Input: part model. Units: mm. Frame: model coordinates. Face numbers are marked on the shaded views. A direction names the side the tool comes from. Coordinates: 2 decimals unless noted, no trailing zeros. Loops run counter-clockwise (first coordinate to the right, second up) from the corner with the lowest first, then second, coordinate; pieces in that order, holes last. Notation, with made-up numbers: (86.25, -4) - (100.25, -4) arc R11 ccw to (100.25, 3) - close; hole circle Ø9 at (6.5, 27.25). An arc over 180 degrees is marked (long way). Write item = value, one per line. Start each with the question number.
from build123d import *

# Parameters (mm, degrees)
SKETCH_1_R          = 14
EXTRUDE_1_DEPTH     = 14
SKETCH_3_R          = 7.5
EXTRUDE_3_DEPTH     = 4
SKETCH_4_R          = 1.75
CUT_EXTRUDE_1_DEPTH = 27.758176321
SKETCH_5_R          = 1
CUT_EXTRUDE_2_DEPTH = 3
SKETCH_6_R          = 1.5
CUT_EXTRUDE_3_DEPTH = 3


with BuildPart() as part:
    # 草图1 → 凸台-拉伸1 (new body)
    with BuildSketch(Plane.XY):
        Circle(SKETCH_1_R)
    extrude(amount=EXTRUDE_1_DEPTH)

    # 草图3 → 凸台-拉伸3 (add)
    with BuildSketch(Plane.XY.offset(14)):
        Circle(SKETCH_3_R)
    extrude(amount=EXTRUDE_3_DEPTH)

    # 草图4 → 切除-拉伸1 (cut, through all)
    with BuildSketch(Plane.XY.offset(18)):
        Circle(SKETCH_4_R)
    extrude(amount=-CUT_EXTRUDE_1_DEPTH, mode=Mode.SUBTRACT)

    # 草图5 → 切除-拉伸2 (cut)
    with BuildSketch(Plane.XY.offset(18)):
        with Locations((0, -6)):
            Circle(SKETCH_5_R)
        with Locations((-6, 0)):
            Circle(SKETCH_5_R)
        with Locations((0, 6)):
            Circle(SKETCH_5_R)
        with Locations((6, 0)):
            Circle(SKETCH_5_R)
    extrude(amount=-CUT_EXTRUDE_2_DEPTH, mode=Mode.SUBTRACT)

    # 草图6 → 切除-拉伸3 (cut)
    with BuildSketch(Plane.XY):
        with Locations((0, 8)):
            Circle(SKETCH_6_R)
        with Locations((-8, 0)):
            Circle(SKETCH_6_R)
        with Locations((0, -8)):
            Circle(SKETCH_6_R)
        with Locations((8, 0)):
            Circle(SKETCH_6_R)
    extrude(amount=CUT_EXTRUDE_3_DEPTH, mode=Mode.SUBTRACT)


solid = part.part
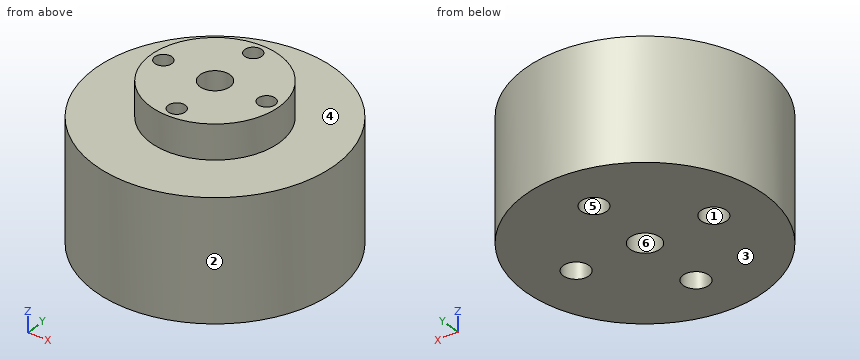
Item 1: Cut plane C-C on z = 1.75. Return loops of the section in (x, y), plus the area to 3 significant figures.
Item 2: Pull-direction query (Y, two-part tool) for the marked faces 1, 2 and 3; classes: pulls with the +Y half, pulls with the -Y half, needs draft (parallel to the pull), parting line crosses it, or undercut.
Item 3: Cut plane D-D on x = 9. Return loops of the section in (y, z), plus the area to 3 significant figures.
Item 4: Pin query (flat end, axial travel): pin 1 (6 mm diameter, centred on x = 8.5, z = 13.5, fed in from -Y); pin 2 (2.5 mm diameter, centred on x = 0, y = 8, fed in from -Z); pin 3 (1.6 mm diameter, centred on x = 0, y = -6, fed in from +Z). Return the tip coordinate at first contact, or that it passes through.
Item 5: Ray query, line 1 (Y direction, x = 0, z = 16.1); line 2 (Y direction, x = 0, z = 6.25); line 3 (Z direction, x = 6, y = 0). Return the intervals inside material, ascending.
Item 6: Cut plane A-A on x = 0. Return loops of the section in (y, z), plus the area to 3 significant figures.
Item 7: Access query for the marked faces 4, 5 and 6. Directions: +Z, -Z, +X, -X, +Y, -Y. A direction counts if a zero-diameter tool reaches every point of the face in a straight line with its end or side. Return the directions, or none.
Recorded:
q1.outline = circle Ø28 at (0, 0); hole circle Ø3 at (-8, 0); hole circle Ø3.5 at (0, 0); hole circle Ø3 at (0, -8); hole circle Ø3 at (0, 8); hole circle Ø3 at (8, 0)
q1.area = 578 mm²
q2.face_1 = undercut
q2.face_2 = parting line crosses it
q2.face_3 = needs draft
q3.outline = (-10.72, 0) - (-1.12, 0) - (-1.12, 3) - (1.12, 3) - (1.12, 0) - (10.72, 0) - (10.72, 14) - (-10.72, 14) - close
q3.area = 294 mm²
q4.pin_1 = -12.87
q4.pin_2 = 3
q4.pin_3 = 15
q5.line_1 = -7.5 to -7, -5 to -1.75, 1.75 to 5, 7 to 7.5
q5.line_2 = -14 to -1.75, 1.75 to 14
q5.line_3 = 0 to 15
q6.outline = (-14, 0) - (-9.5, 0) - (-9.5, 3) - (-6.5, 3) - (-6.5, 0) - (-1.75, 0) - (-1.75, 18) - (-5, 18) - (-5, 15) - (-7, 15) - (-7, 18) - (-7.5, 18) - (-7.5, 14) - (-14, 14) - close; (1.75, 0) - (6.5, 0) - (6.5, 3) - (9.5, 3) - (9.5, 0) - (14, 0) - (14, 14) - (7.5, 14) - (7.5, 18) - (7, 18) - (7, 15) - (5, 15) - (5, 18) - (1.75, 18) - close
q6.area = 359 mm²
q7.face_4 = +Z
q7.face_5 = -Z
q7.face_6 = +Z, -Z
